from build123d import *

# Parameters (mm, degrees)
F0_R     = 24.5
F1_DEPTH = 10.5
F2_T     = -2.5
F5_R     = 5


with BuildPart() as f1:
    # F0 (on Top) → F1 (new body, symmetric)
    with BuildSketch(Plane.XY):
        Circle(F0_R)
    extrude(amount=F1_DEPTH, both=True)

    # F2
    f2_openings = [f1.faces().sort_by_distance(p)[0] for p in [
        (0, 0, 10.5),
    ]]
    offset(amount=F2_T, openings=f2_openings)

    # F3 (on Front) → F4 (revolve, cut)
    with BuildSketch(Plane.XZ):
        with BuildLine():
            Line((-22, 2.023608), (-22, 8.213608))
            ThreePointArc((-22, 8.213608), (-23.237886, 5.118608), (-22, 2.023608))
        make_face()
    revolve(axis=Axis((0, 0, 3.342178), (0, 0, -1)), mode=Mode.SUBTRACT)

    # F5
    f5_edges = [f1.edges().sort_by_distance(p)[0] for p in [
        (-24.5, 0, -10.5),
    ]]
    fillet(f5_edges, radius=F5_R)


solid = f1.part
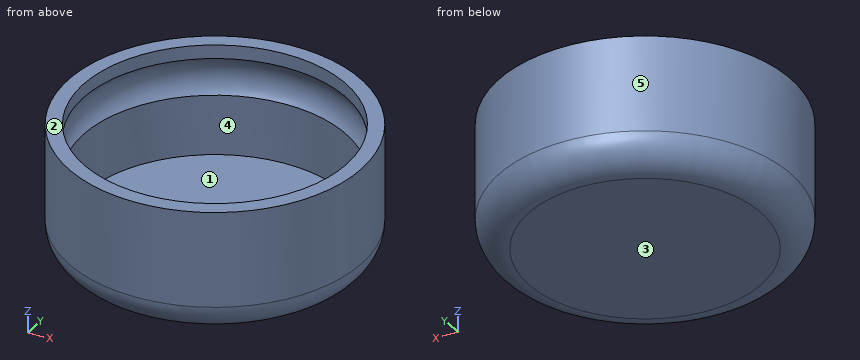
Can you work these out from the model? Positions are in its coordinate system, mm. Face numbers are marked on the shaded views. A direction names the side the tool comes from. Coordinates: 2 decimals unless noted, no trailing zeros. Write each loop counter-clockwise with the first axis right and the second up, starting at its lowest first coordinate (ties: lowest second). Pieces come first, ordered by that corner, then holes. Notation, with made-up numbers: M -35.5,-19.5 L 1.5,-19.5 A17 ccw 1.5,10.5 Z; hole C 25,56.25 d6. An arc over 180 degrees is marked long. Use one line per item in the form item = value.
Q1. If we section it at A-A (x = 0): Write out the boundary of the cut face in (y, z), then the cut area to 3 significant figures.
Model answer:
outline = M -24.5,-5.5 A5 ccw -19.5,-10.5 L 19.5,-10.5 A5 ccw 24.5,-5.5 L 24.5,10.5 L 22,10.5 L 22,8.21 A4.49 cw 22,2.02 L 22,-8 L -22,-8 L -22,2.02 A4.49 cw -22,8.21 L -22,10.5 L -24.5,10.5 Z
area = 194 mm^2
Q2. We'd pull the mould along X, two halves only. Please class the marked faces 3, 4 and 5: +X half, -X half, draft (parallel to the pull), parting line (faces both ways), or undercut.
Model answer:
face_3 = draft
face_4 = undercut
face_5 = parting line
Q3. I need wall thicknesses on line 1 along Y through (x, z) = (0, -2); line 2 along Z through (x, y) = (-8.5, -2); line 3 along X through (y, z) = (14.5, -3.5). Which ranges of each line are inside material? Lowest first, please. Write a range as from..to.
Model answer:
line_1 = -24.5..-22, 22..24.5
line_2 = -10.5..-8
line_3 = -19.75..-16.55, 16.55..19.75
Q4. If we section it at C-C (z = -2.5): Write out the boundary of the cut face in (x, y), then the cut area to 3 significant figures.
Model answer:
outline = C 0,0 d49; hole C 0,0 d44
area = 365 mm^2
Q5. For P1, Ø5, axis at x = -18, z = -3, coming from the -Y side; P2, Ø10, axis at y = -16.5, z = -1.5, coming from the -X side; P3, Ø2, axis at x = -17, y = 18.5, coming from the -Z side, each with a flat end and sliding along its axis, tell me the tip position at first contact or that it passes through.
Model answer:
P1 = -18.97
P2 = -21.63
P3 = -7.4
Q6. If we section it at D-D (z = -6.5): Write out the boundary of the cut face in (x, y), then the cut area to 3 significant figures.
Model answer:
outline = C 0,0 d48.8; hole C 0,0 d44
area = 350 mm^2
Q7. For the marked faces 1 and 2, which set-ups out of +Z, -Z, +X, -X, +Y, -Y let a thin tool reach every point of the face, with its end or its side?
Model answer:
face_1 = +Z
face_2 = +Z, +X, -X, +Y, -Y
